Autodesk Inventor part; units mm, degrees
ref_plane "YZ Plane" through (0, 0, 0) normal (1, 0, 0) x (0, 1, 0)
ref_plane "XZ Plane" through (0, 0, 0) normal (0, 1, 0) x (-1, 0, 0)
ref_plane "XY Plane" through (0, 0, 0) normal (0, 0, 1) x (1, 0, 0)
sketch "スケッチ1" plane through (0, 0, 0) normal (0, 0, 1) x (1, 0, 0)
  circle A0 centre (0, 0) radius 4
  dimension "d0" = 8
extrude "押し出し1" add sketch "スケッチ1" along normal blind 1
sketch "スケッチ2" plane through (0, 0, 1) normal (0, 0, 1) x (1, 0, 0)
  circle A0 centre (0, 0) radius 2.5
  dimension "d3" = 5
extrude "押し出し2" add sketch "スケッチ2" along normal blind 5
sketch "スケッチ3" plane through (0, 0, 6) normal (0, 0, 1) x (1, 0, 0)
  point P0 (0, 0)
  point P1 (0, 0)
hole "穴1" at (0, 0, 6) direction (0, 0, -1) diameter 3 end through all
properties part number "RD016"
Model file for the job. Use its own axes, mm. A direction names the side the tool comes from. Give positions to 0.01 mm unless a question says otherwise; leave off trailing zeros. Write each loop counter-clockwise with the first axis right and the second up, starting at its lowest first coordinate (ties: lowest second). Pieces come first, ordered by that corner, then holes. Notation, with made-up numbers: M 83,56.25 L 137,56.25 A26 cw 137,94.25 Z; hole C 50.5,74.5 d11. An arc over 180 degrees is marked long. One line per item, written item: value. Start each with the question number.
Q1. 3-axis set-ups, long thin cutter, end or side, ignore diameter. For faces 4 (the flat face through (2, 0, 0)), 5 (the cylindrical face through (-0.54, 2.44, 3.46)): which of +Z, -Z, +X, -X, +Y, -Y reach the whole face in a straight line?
Q2. Saw through at D-D, the plane y = -2. Write the cut outline in (x, z), plus the area to 3 significant figures.
Q3. Saw through at C-C, the plane z = 2.75. Write the cut outline in (x, y), plus the area to 3 significant figures.
Q4. Probe probe 1 along Y at (x, z) = (0, 4.7); probe 2 along Z at (x, y) = (-0.5, -3.5); probe 3 along X at (y, z) = (0.5, 2.85). List the from-to ranges inside material, lowest first. Write a range as [from, to].
Q5. Drop flat-ended pins along their axis: pin 1 Ø3 at (y, z) = (-1.5, 4.5) entering from +X; pin 2 Ø3 at (y, z) = (2, 2) entering from -X. Give the stop position or say it passes through.
Q6. Two-plate mould, pull along X, no slides. Class faces 1 (the cylindrical face through (-0.867, 3.905, 0.493)), 2 (the cylindrical face through (-0.07, 1.5, 2.96)), 3 (the flat face through (2, 0, 6)): +X half, -X half, draft (parallel to the pull), parting line (faces both ways), or undercut.
Q7. Saw through at A-A, the plane x = 0. Write the cut outline in (y, z), plus the area to 3 significant figures.
Output values:
1. face 4: -Z, +X, -X, +Y, -Y
1. face 5: +Z
2. outline: M -3.46,0 L 3.46,0 L 3.46,1 L 1.5,1 L 1.5,6 L -1.5,6 L -1.5,1 L -3.46,1 Z
2. area: 21.9 mm²
3. outline: C 0,0 d5; hole C 0,0 d3
3. area: 12.6 mm²
4. probe 1: y = [-2.5, -1.5], [1.5, 2.5]
4. probe 2: z = [0, 1]
4. probe 3: x = [-2.45, -1.41], [1.41, 2.45]
5. pin 1: stops at x = 2.5
5. pin 2: stops at x = -3.9
6. face 1: parting line
6. face 2: undercut
6. face 3: draft
7. outline: M -4,0 L -1.5,0 L -1.5,6 L -2.5,6 L -2.5,1 L -4,1 Z; M 1.5,0 L 4,0 L 4,1 L 2.5,1 L 2.5,6 L 1.5,6 Z
7. area: 15.0 mm²
